```python
from build123d import *

# Parameters (mm, degrees)
RESSALTO_EXTRUS_O1_DEPTH = 216
FILETE1_R                = 0.5
ESBO_O2_R                = 1.5
CORTE_EXTRUS_O1_DEPTH    = 217


with BuildPart() as part:
    # Esboço1 → Ressalto-extrusão1 (new body)
    with BuildSketch(Plane(origin=(0, 0, 0), x_dir=(-1, 0, 0), z_dir=(0, 0, -1))):
        Polygon((67.502122675, -1.443375673), (70.002122675, -2.886751346), (72.502122675, -1.443375673), (72.502122675, 1.443375673), (70.002122675, 2.886751346), (67.502122675, 1.443375673), align=None)
    extrude(amount=-RESSALTO_EXTRUS_O1_DEPTH)

    # Filete1
    filete1_edges = [part.edges().sort_by_distance(p)[0] for p in [
        (-71.252122675, -2.165063509, 216),
        (-72.502122675, 0, 216),
        (-71.252122675, 2.165063509, 216),
        (-68.752122675, 2.165063509, 216),
        (-67.502122675, 0, 216),
        (-68.752122675, 2.165063509, 0),
        (-71.252122675, 2.165063509, 0),
        (-72.502122675, 0, 0),
        (-71.252122675, -2.165063509, 0),
        (-68.752122675, -2.165063509, 0),
        (-67.502122675, 0, 0),
        (-68.752122675, -2.165063509, 216),
    ]]
    fillet(filete1_edges, radius=FILETE1_R)

    # Esboço2 → Corte-extrusão1 (cut, through all)
    with BuildSketch(Plane.XY.offset(216)):
        with Locations((-70.002122675, 0)):
            Circle(ESBO_O2_R)
    extrude(amount=-CORTE_EXTRUS_O1_DEPTH, mode=Mode.SUBTRACT)


solid = part.part
```
Model file for the job. Use its own axes, mm. Give positions to 0.01 mm unless a question says otherwise; leave off trailing zeros. Order: outer loops, then holes, each group sorted by start corner. A loop starts at its lowest first (then second) coordinate and runs counter-clockwise, first axis right, second up.
1) Pin check, flat tips, straight feed: pin 1 (1 mm diameter, centred on x = -71, z = 100, fed in from +Y); pin 2 (1.5 mm diameter, centred on x = -71, z = 77, fed in from -Y); pin 3 (1.5 mm diameter, centred on x = -72, z = 183.5, fed in from +Y). Stop position of each tip, or through.
2) Wall check: probe 1 along X at (y, z) = (-0.1, 207); probe 2 along Y at (x, z) = (-70.05, 56); probe 3 along Y at (x, z) = (-71.35, 146.5). Give the ranges that are in metal, low to high.
3) Saw through at B-B, the plane z = 19. Write the cut outline in (x, y), then the cut area to 3 significant figures.
4) Saw through at A-A, the plane y = 0. Write the cut outline in (x, z), then the cut area to 3 significant figures.
Computed:
1. pin 1: stops at y = 2.6
1. pin 2: stops at y = -2.74
1. pin 3: stops at y = 2.17
2. probe 1: x = -72.5 to -71.5, -68.51 to -67.5
2. probe 2: y = -2.86 to -1.5, 1.5 to 2.86
2. probe 3: y = -2.11 to -0.66, 0.66 to 2.11
3. outline: (-72.5, -1.44) - (-70, -2.89) - (-67.5, -1.44) - (-67.5, 1.44) - (-70, 2.89) - (-72.5, 1.44) - close; hole circle Ø3 at (-70, 0)
3. area: 14.6 mm2
4. outline: (-72.5, 0.5) arc R0.5 ccw to (-72, 0) - (-71.5, 0) - (-71.5, 216) - (-72, 216) arc R0.5 ccw to (-72.5, 215.5) - close; (-68.5, 0) - (-68, 0) arc R0.5 ccw to (-67.5, 0.5) - (-67.5, 215.5) arc R0.5 ccw to (-68, 216) - (-68.5, 216) - close
4. area: 432 mm2
